Autodesk Inventor part; units mm, degrees
ref_plane "Work Plane1" through (0, 0, -152.4) normal (0, 0, 1) x (1, 0, 0)
ref_plane "YZ Plane" through (0, 0, 0) normal (1, 0, 0) x (0, 1, 0)
ref_plane "XZ Plane" through (0, 0, 0) normal (0, 1, 0) x (-1, 0, 0)
sketch "Sketch1" plane through (0, 0, 0) normal (0, 0, 1) x (1, 0, 0)
  circle A0 centre (0, 0) radius 304.8
  dimension "d0" = 609.6
extrude "Extrusion1" add sketch "Sketch1" against normal blind 1828.8
ref_plane "Work Plane1" through (0, 0, -152.4) normal (0, 0, 1) x (1, 0, 0)
sketch "Sketch2" plane through (0, 0, -152.4) normal (0, 0, 1) x (1, 0, 0)
  circle A0 centre (0, 0) radius 190.5
  dimension "d4" = 381
extrude "Extrusion2" add sketch "Sketch2" along normal blind 609.6 draft 20
sketch "Sketch4" plane through (0, 0, -152.4) normal (0, 0, 1) x (1, 0, 0)
  circle A0 centre (0, 0) radius 38.1
  dimension "d7" = 76.2
extrude "Extrusion3" cut sketch "Sketch4" along normal blind 609.6 draft 25
properties part number "sep_motors"
The listing builds one solid part. Answer for the finished solid, in the listing's coordinates (mm). A direction names the side the tool comes from. Coordinates: 2 decimals unless noted, no trailing zeros. Write each loop counter-clockwise with the first axis right and the second up, starting at its lowest first coordinate (ties: lowest second). Pieces come first, ordered by that corner, then holes. Notation, with made-up numbers: (2, 12) - (50, 12) arc R18 ccw to (50, 46) - close; hole circle Ø1 at (6.5, 16). An arc over 180 degrees is marked (long way). One line per item, written item: value.
1) Consider line 1 along Y through (x, z) = (-121.5, 334.5); line 2 along X through (y, z) = (2, -319); line 3 along Y through (x, z) = (123.5, 142.5). Determine where each line is inside the solid, lowest interval first. Write a range as from..to.
Geometry check:
line 1: y = -347.06..-235.67, 235.67..347.06
line 2: x = -304.79..304.79
line 3: y = -271.02..-124.85, 124.85..271.02
2) A tool of negligible diameter and unlimited length cuts with its end or side. For faces 5 (the cylindrical face through (-241.879, -185.466, -901.598)), 6 (the flat face through (-4, 4, -1828.8)), from which of +Z, -Z, +X, -X, +Y, -Y can it reach the whole face along a straight path? Write none if from no direction.
Geometry check:
face 5: -Z
face 6: -Z, +X, -X, +Y, -Y
3) Find section C-C (z = -1652.5). Give the vertices of the cut face in (x, y), and give its area (3 significant figures).
Geometry check:
outline: circle Ø609.6 at (0, 0)
area: 292,000 mm2
4) For a pull along Y with two mould halves and no side action, classify faces 1 (the conical face through (-232.8, -178.5, 130.2)), 2 (the flat face through (-205, 137, 0)), 3 (the flat face through (-1, 1, -152.4)), 4 (the conical face through (-119.539, -91.66, 88.934)) as pulls with the +Y half, pulls with the -Y half, needs draft (parallel to the pull), parting line crosses it, or undercut.
Geometry check:
face 1: parting line crosses it
face 2: needs draft
face 3: undercut
face 4: undercut
5) Find section D-D (z = 278). Give the vertices of the cut face in (x, y), and give its area (3 significant figures).
Geometry check:
outline: circle Ø694.31 at (0, 0); hole circle Ø477.6 at (0, 0)
area: 199,000 mm2
6) Each of these flat-tipped pins is pushed along its axis until it touches: pin 1 Ø12 at (y, z) = (-83.5, -319.5) entering from -X; pin 2 Ø8 at (x, z) = (-166, -1211.5) entering from +Y; pin 3 Ø10 at (y, z) = (-163, -220.5) entering from +X. Where does it stop, or does it pass through?
Geometry check:
pin 1: stops at x = -294.78
pin 2: stops at y = 258.18
pin 3: stops at x = 260.65
7) Find section A-A (y = 0). Give the vertices of the cut face in (x, z).
Geometry check:
outline: (-412.38, 457.2) - (-245.97, 0) - (-304.8, 0) - (-304.8, -1828.8) - (304.8, -1828.8) - (304.8, 0) - (245.97, 0) - (412.38, 457.2) - (322.36, 457.2) - (38.1, -152.4) - (-38.1, -152.4) - (-322.36, 457.2) - close
